Geometry check sheet. Reference: drawing and pictorial views, mm from the part's lowest x, y, z. Coordinates: 2 decimals unless noted, no trailing zeros. Order: outer loops, then holes, each group sorted by start corner. A loop starts at its lowest first (then second) coordinate and runs counter-clockwise, first axis right, second up. Notation, with made-up numbers: M 57.5,-34.5 L 74.5,-34.5 A23 ccw 74.5,-12.5 Z; hole C -38,27.25 d3. An arc over 180 degrees is marked long. Return JSON: item names as keys, results as strings.
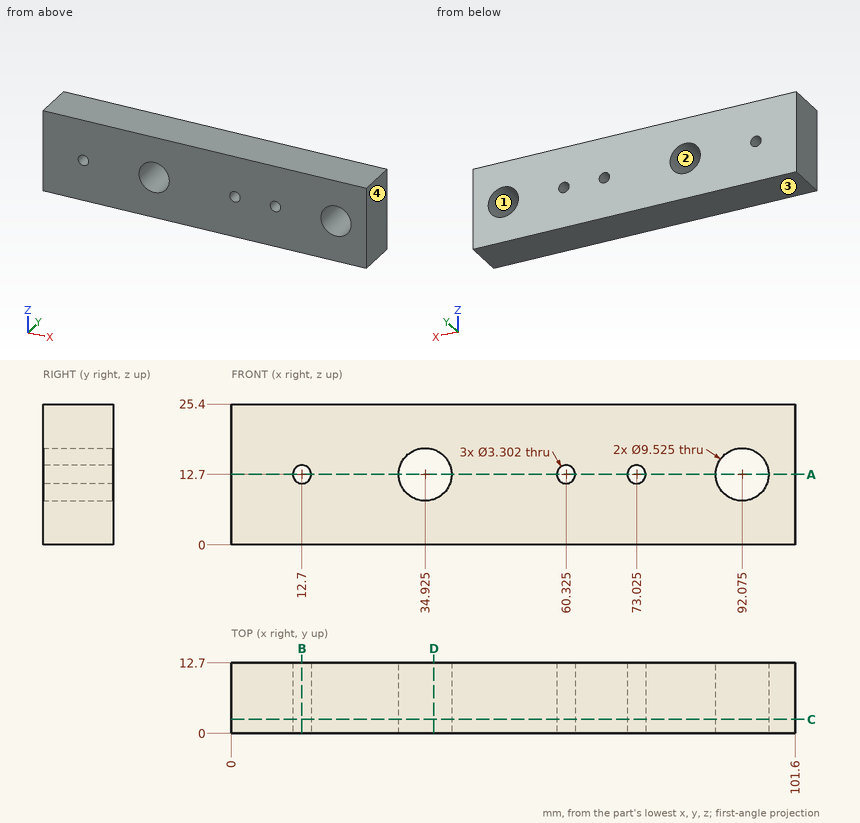
Q1. Go/stop test with a flat-tipped pin: pin 1 (7.5 mm diameter, centred on x = 34.925, z = 12.7, fed in from -Y). Record where the tip stops, or that it passes through.
Values:
{"pin 1": "through"}
Q2. Material ranges on line 1 along X through (y, z) = (10, 12.7); line 2 along X through (y, z) = (6.25, 13.5); line 3 along Z through (x, y) = (12.7, 6.5), recorded low to high.
Values:
{"line 1": "0 to 11.05, 14.35 to 30.16, 39.69 to 58.67, 61.98 to 71.37, 74.68 to 87.31, 96.84 to 101.6", "line 2": "0 to 11.26, 14.14 to 30.23, 39.62 to 58.88, 61.77 to 71.58, 74.47 to 87.38, 96.77 to 101.6", "line 3": "0 to 11.05, 14.35 to 25.4"}
Q3. Cross-section at B-B, the plane x = 12.7. Record the boundary of the cut face in (y, z).
Values:
{"outline": "M 0,0 L 12.7,0 L 12.7,11.05 L 0,11.05 Z; M 0,14.35 L 12.7,14.35 L 12.7,25.4 L 0,25.4 Z"}
Q4. Cross-section at A-A, the plane z = 12.7. Record the boundary of the cut face in (x, y), and give its area (3 significant figures).
Values:
{"outline": "M 0,0 L 11.05,0 L 11.05,12.7 L 0,12.7 Z; M 14.35,0 L 30.16,0 L 30.16,12.7 L 14.35,12.7 Z; M 39.69,0 L 58.67,0 L 58.67,12.7 L 39.69,12.7 Z; M 61.98,0 L 71.37,0 L 71.37,12.7 L 61.98,12.7 Z; M 74.68,0 L 87.31,0 L 87.31,12.7 L 74.68,12.7 Z; M 96.84,0 L 101.6,0 L 101.6,12.7 L 96.84,12.7 Z", "area": "923 mm^2"}
Q5. Cross-section at D-D, the plane x = 36.5. Record the boundary of the cut face in (y, z), and give its area (3 significant figures).
Values:
{"outline": "M 0,0 L 12.7,0 L 12.7,8.21 L 0,8.21 Z; M 0,17.19 L 12.7,17.19 L 12.7,25.4 L 0,25.4 Z", "area": "208 mm^2"}
Q6. Cross-section at C-C, the plane y = 2.5. Record the boundary of the cut face in (x, z) (1 decimal), and give its area (3 significant figures).
Values:
{"outline": "M 0,0 L 101.6,0 L 101.6,25.4 L 0,25.4 Z; hole C 12.7,12.7 d3.3; hole C 34.9,12.7 d9.5; hole C 60.3,12.7 d3.3; hole C 73,12.7 d3.3; hole C 92.1,12.7 d9.5", "area": "2,410 mm^2"}
Q7. Draft check along X on the marked faces 1, 2, 3 and 4. Enter one of: pulls with the +X half, pulls with the -X half, needs draft (parallel to the pull), parting line crosses it, or undercut.
Values:
{"face 1": "undercut", "face 2": "undercut", "face 3": "needs draft", "face 4": "pulls with the +X half"}
